For this review, take the finished solid that the model builds, in its own axes (mm). Face numbers are marked on the shaded views. A direction names the side the tool comes from. Round coordinates to 2 decimals unless told otherwise and drop trailing zeros. Order: outer loops, then holes, each group sorted by start corner. A loop starts at its lowest first (then second) coordinate and runs counter-clockwise, first axis right, second up. Notation, with made-up numbers: (3, 36) - (43, 36) arc R19 cw to (43, 72) - close; hole circle Ø1 at (13.5, 13). An arc over 180 degrees is marked (long way). Write each question's results on one line, items separated by ' | '. Start each with the question number.
(1) For L1, parallel to X at y = 56.5, z = -39 (3 decimals); L2, parallel to Y at x = 6, z = -6, list the stretches that pass through material, from the lowest coordinate up. Write a range as from..to.
(2) Take a section at B-B, the plane y = 52. Give the boundary of the cut face in (x, z) (3 decimals).
(3) For the marked faces 1 and 2, list the 3-axis set-ups (+Z, -Z, +X, -X, +Y, -Y) from which the entire face can be reached by the end or side of a thin tool; tool diameter is ignored.
(4) Insertion check: pin 1 Ø24.5 at (y, z) = (25.5, -3) entering from +X (3 decimals); pin 2 Ø19 at (x, z) = (24, 1) entering from +Y (3 decimals). Each pin has a flat end and moves straight along its axis. Give the tip position at first contact, or say it passes through.
```python
from build123d import *

# Parameters (mm, degrees)
BASESTEELANGLE_DEPTH = 63.5


with BuildPart() as part:
    # Sketch1 → BaseSteelAngle (new body, symmetric)
    with BuildSketch(Plane.XY):
        with BuildLine():
            Line((0, 0), (0, 60.325))
            Line((0, 60.325), (0.00508, 60.325))
            ThreePointArc((0.00508, 60.325), (2.246551928, 59.396551928), (3.175, 57.15508))
            Line((3.175, 57.15508), (3.175, 7.9375))
            ThreePointArc((3.175, 7.9375), (4.569903955, 4.569903955), (7.9375, 3.175))
            Line((7.9375, 3.175), (31.75508, 3.175))
            ThreePointArc((31.75508, 3.175), (33.996551928, 2.246551928), (34.925, 0.00508))
            Line((34.925, 0.00508), (34.925, 0))
            Line((34.925, 0), (0, 0))
        make_face()
    extrude(amount=BASESTEELANGLE_DEPTH, both=True)


solid = part.part
```
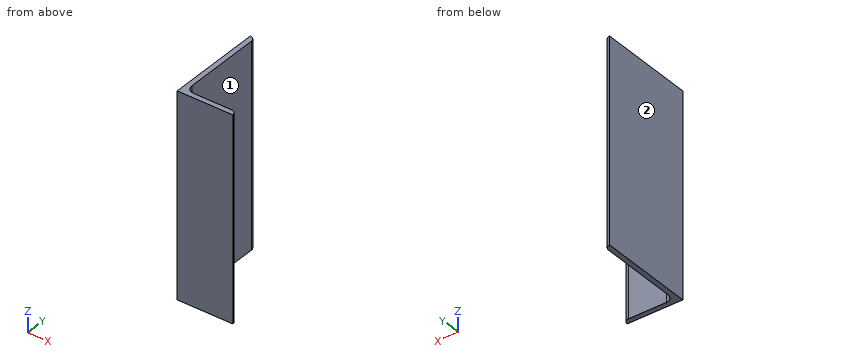
Results below:
1) L1: x = 0..3.175 | L2: y = 0..3.59
2) outline: (0, -63.5) - (3.175, -63.5) - (3.175, 63.5) - (0, 63.5) - close
3) face 1: +Z, -Z, +X, +Y | face 2: +Z, -Z, -X, +Y, -Y
4) pin 1: stops at x = 3.175 | pin 2: stops at y = 3.175
